Here's how the part is built. I have some questions about the finished solid (model axes, mm). Face numbers are marked on the shaded views. A direction names the side the tool comes from. Give positions to 0.01 mm unless a question says otherwise; leave off trailing zeros. Write each loop counter-clockwise with the first axis right and the second up, starting at its lowest first coordinate (ties: lowest second). Pieces come first, ordered by that corner, then holes. Notation, with made-up numbers: (70.25, 74) -> (129.25, 74) arc R14 ccw to (129.25, 82) -> close; hole circle Ø10 at (72, -22). An arc over 180 degrees is marked (long way). Use one line per item in the form item = value.
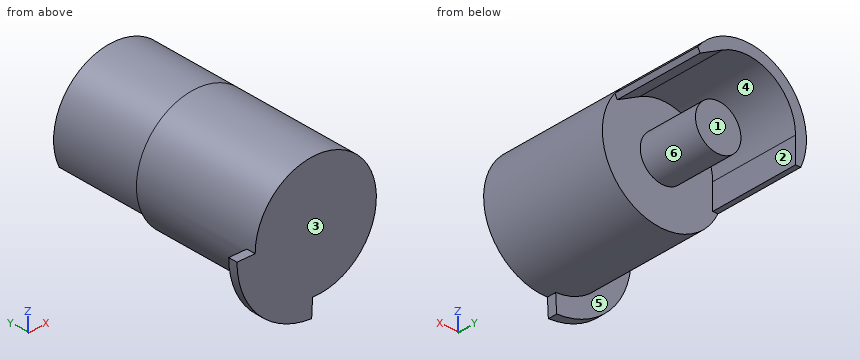
```python
from build123d import *

# Parameters (mm, degrees)
SKETCH1_R           = 10
SKETCH1_R_2         = 8.018181818
BOSS_EXTRUDE1_DEPTH = 21.5
BOSS_EXTRUDE2_DEPTH = 15
SKETCH3_R           = 3.75
BOSS_EXTRUDE3_DEPTH = 10
BOSS_EXTRUDE4_DEPTH = 1.5


with BuildPart() as part:
    # Sketch1 → Boss-Extrude1 (new body)
    # profile 1 of 2: a face of its own
    with BuildSketch(Plane(origin=(0, 0, 0), x_dir=(1, 0, 0), z_dir=(0, 1, 0))):
        with Locations(Location((0, 0, 0), (0, 0, 270))):
            Circle(SKETCH1_R)
        Circle(SKETCH1_R_2, mode=Mode.SUBTRACT)
    # profile 2 of 2: a face of its own
    with BuildSketch(Plane(origin=(0, 0, 0), x_dir=(1, 0, 0), z_dir=(0, 1, 0))):
        Circle(SKETCH1_R_2)
    extrude(amount=BOSS_EXTRUDE1_DEPTH)

    # Sketch2 → Boss-Extrude2 (add)
    with BuildSketch(Plane(origin=(0, 21.5, 0), x_dir=(1, 0, 0), z_dir=(0, 1, 0))):
        with BuildLine():
            ThreePointArc((3.849666815, -7.240170261), (-4.223312214, -7.028771866), (-8.2, 0))
            Line((-8.2, 0), (-8.2, 4.223635209))
            Line((-8.2, 4.223635209), (-9.064265311, 4.223635209))
            ThreePointArc((-9.064265311, 4.223635209), (-5.183292284, -8.551811568), (7.938142814, -6.081602475))
            Line((7.938142814, -6.081602475), (7.538265506, -5.315317068))
            Line((7.538265506, -5.315317068), (3.849666815, -7.240170261))
        make_face()
    extrude(amount=BOSS_EXTRUDE2_DEPTH)

    # Sketch3 → Boss-Extrude3 (add)
    with BuildSketch(Plane(origin=(0, 21.5, 0), x_dir=(1, 0, 0), z_dir=(0, 1, 0))):
        with Locations(Location((0, 0, 0), (0, 0, 270))):
            Circle(SKETCH3_R)
    extrude(amount=BOSS_EXTRUDE3_DEPTH)

    # Sketch4 → Boss-Extrude4 (add)
    with BuildSketch(Plane(origin=(0, 0, 0), x_dir=(1, 0, 0), z_dir=(0, 1, 0))):
        with BuildLine():
            ThreePointArc((-0.680367431, 12.982183952), (-9.429866823, 8.948609484), (-13, 0))
            Line((-13, 0), (-10, 0))
            ThreePointArc((-10, 0), (-9.99657325, 0.261769483), (-9.986295348, 0.523359562))
            ThreePointArc((-9.986295348, 0.523359562), (-7.071067812, 7.071067812), (-0.523359562, 9.986295348))
            Line((-0.523359562, 9.986295348), (-0.680367431, 12.982183952))
        make_face()
    extrude(amount=BOSS_EXTRUDE4_DEPTH)


solid = part.part
```
Q1. Will these pins go through, and if not, where does the flat tip stop? pin 1 Ø2 at (y, z) = (19.5, 7) entering from +X; pin 2 Ø5 at (x, z) = (-1.5, -8.5) entering from +Y; pin 3 Ø6 at (y, z) = (26, -2) entering from -X.
Result set:
pin_1 = 8
pin_2 = 21.5
pin_3 = -10
Q2. I want a section at B-B, the plane x = 0. Write out the boundary of the cut face in (y, z).
Result set:
outline = (0, -10) -> (21.5, -10) -> (21.5, -3.75) -> (31.5, -3.75) -> (31.5, 3.75) -> (21.5, 3.75) -> (21.5, 8.2) -> (36.5, 8.2) -> (36.5, 10) -> (0, 10) -> close
Q3. If we mould it in two halves opening along X, with no side actions, what happens to the marked faces 4, 5 and 6? For each: +X half, -X half, draft (parallel to the pull), parting line (faces both ways), or undercut.
Result set:
face_4 = undercut
face_5 = draft
face_6 = undercut
Q4. I want a section at C-C, the plane z = -2.75. Write out the boundary of the cut face in (x, y).
Result set:
outline = (-12.71, 0) -> (9.61, 0) -> (9.61, 21.5) -> (2.55, 21.5) -> (2.55, 31.5) -> (-2.55, 31.5) -> (-2.55, 21.5) -> (-8.2, 21.5) -> (-8.2, 36.5) -> (-9.61, 36.5) -> (-9.61, 1.5) -> (-12.71, 1.5) -> close
Q5. Which directions (+Z, -Z, +X, -X, +Y, -Y) give clear straight access to the entire face, cutting with the end or side of a thin tool? Please do the marked faces 1, 2 and 3.
Result set:
face_1 = -Z, +X, +Y
face_2 = -Z, +Y
face_3 = +Z, -Z, +X, -X, -Y
Q6. I want a section at D-D, the plane y = 33. Write out the boundary of the cut face in (x, z), and give its area (3 significant figures).
Result set:
outline = (-9.06, -4.22) -> (-8.2, -4.22) -> (-8.2, 0) arc R8.2 cw to (3.85, 7.24) -> (7.54, 5.32) -> (7.94, 6.08) arc R10 ccw to start
area = 46.2 mm2
Q7. If I drill on line 1 along Y through (x, z) = (5.75, 6); line 2 along X through (y, z) = (27, 7); line 3 along Y through (x, z) = (-3, -10.5), over which ranges is the centre line in solid material (lowest first)? Write a range as from..to.
Result set:
line_1 = 0..21.5
line_2 = -7.14..-4.27, 4.31..7.14
line_3 = 0..1.5
Q8. I want a section at A-A, the plane y = 22. Write out the boundary of the cut face in (x, z), and give its area (3 significant figures).
Result set:
outline = (-9.06, -4.22) -> (-8.2, -4.22) -> (-8.2, 0) arc R8.2 cw to (3.85, 7.24) -> (7.54, 5.32) -> (7.94, 6.08) arc R10 ccw to start; circle Ø7.5 at (0, 0)
area = 90.4 mm2
